Autodesk Inventor part; units mm, degrees
ref_plane "Work Plane1" through (35, 60, 0) normal (1, 0, 0) x (0, 1, 0)
ref_plane "Work Plane2" through (35, 5, 0) normal (1, 0, 0) x (0, 1, 0)
ref_plane "Work Plane3" through (35, 20, 0) normal (1, 0, 0) x (0, 1, 0)
sketch "Sketch1" plane through (0, 0, 0) normal (0, 0, 1) x (1, 0, 0)
  line L0 (0, 0) -> (0, 70)
  line L1 (0, 70) -> (-35, 70)
  line L2 (-35, 70) -> (-35, 5)
  line L3 (0, 0) -> (-32.5, 0)
  arc A0 (-35, 5) -> (-32.5, 0) centre (-28.75, 5) ccw
  dimension "d0" = 70
  dimension "d1" = 35
  dimension "d2" = 65
  dimension "d3" = 32.5
revolve "Revolution1" add sketch "Sketch1" angle 360 about axis through (0, 0, 0) along (0, 1, 0)
shell "Shell1" thickness 3 removed faces 1 at (-0.2748, 70, -9.3581)
sketch "Sketch2" plane through (0, 0, 0) normal (0, 0, 1) x (1, 0, 0)
  line L0 (35, 60) -> (60, 60)
  line L1 (35, 20) -> (64.0906, 49.6106)
  line L2 (35, 5) -> (35, 70)
  arc A0 (64.0906, 49.6106) -> (60, 60) centre (60, 54) ccw
ref_plane "Work Plane1" through (35, 60, 0) normal (1, 0, 0) x (0, 1, 0)
sketch "Sketch3" plane through (35, 60, 0) normal (1, 0, 0) x (0, 1, 0)
  ellipse E0 centre (0, 0) end of major axis (0, -6) minor radius 2
  point P0 (-60, 0)
ref_plane "Work Plane2" through (35, 5, 0) normal (1, 0, 0) x (0, 1, 0)
sketch "Sketch4" plane through (35, 5, 0) normal (1, 0, 0) x (0, 1, 0)
  point P0 (-5, 0)
ref_plane "Work Plane3" through (35, 20, 0) normal (1, 0, 0) x (0, 1, 0)
sketch "Sketch5" plane through (35, 20, 0) normal (1, 0, 0) x (0, 1, 0)
  ellipse E0 centre (0, 0) end of major axis (0, -5) minor radius 3
  point P0 (-20, 0)
sweep "Sweep1" add profiles "Sketch3" path "Sketch2" path curves L0 A0 L1
fillet "Fillet1" radius 2 2 edges at (35, 70, 0) (32, 70, 0)
sketch "Sketch6" plane through (0, 0, 0) normal (0, -1, 0) x (1, 0, 0)
  circle A0 centre (0, 0) radius 31
  circle A1 centre (0, 0) radius 32.5
  dimension "d34" = 62
  dimension "d35" = 65
extrude "Extrusion1" add sketch "Sketch6" along normal blind 2 contours A0 | A1
properties part number "Lab No. 2"
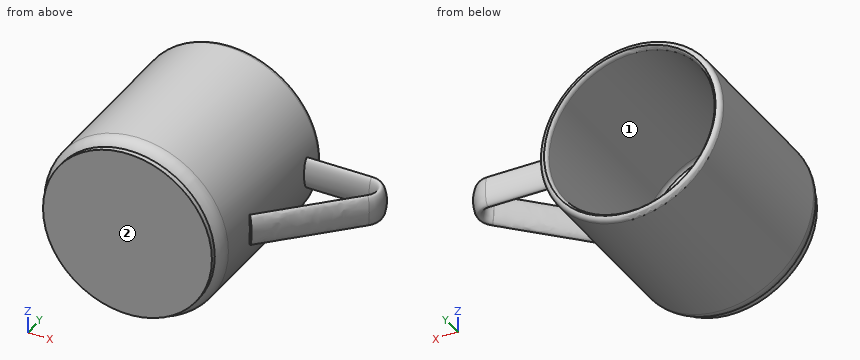
Can you work these out from the model? Positions are in its coordinate system, mm. Face numbers are marked on the shaded views. Give positions to 0.01 mm unless a question says otherwise; leave off trailing zeros. Loops run counter-clockwise (first coordinate to the right, second up) from the corner with the lowest first, then second, coordinate; pieces in that order, holes last. Notation, with made-up numbers: (84.5, 3.25) -> (121.5, 3.25) arc R27 ccw to (121.5, 37.25) -> close; hole circle Ø11 at (26.5, 89). An arc over 180 degrees is marked (long way). Return JSON: item names as keys, results as strings.
Q1. We'd pull the mould along X, two halves only. Please class the marked faces 1 and 2: released by +X, released by -X, zero draft, split by the parting line, or undercut.
Checks:
{"face 1": "undercut", "face 2": "zero draft"}
Q2. I want a section at A-A, the plane x = 0. List the corners of the cut face in (y, z) for me, then the cut area to 3 significant figures.
Checks:
{"outline": "(-2, -32.5) -> (0, -32.5) arc R6.25 ccw to (5, -35) -> (68, -35) arc R2 ccw to (70, -33) arc R2 ccw to (68.27, -32) -> (5, -32) arc R3.25 cw to (3, -31.31) -> (3, 31.31) arc R3.25 cw to (5, 32) -> (68.27, 32) arc R2 ccw to (70, 33) arc R2 ccw to (68, 35) -> (5, 35) arc R6.25 ccw to (0, 32.5) -> (-2, 32.5) -> close", "area": "733 mm2"}
Q3. For pin 1 Ø6 at (x, z) = (48, 0) entering from +Y; pin 2 Ø5 at (y, z) = (47, -2.5) entering from -X; pin 3 Ø5 at (x, y) = (-19.5, 48) entering from -Z; pin 4 Ø5 at (y, z) = (5.5, -18) entering from +X, each with a flat end and sliding along its axis, tell me the tip position at first contact or that it passes through.
Checks:
{"pin 1": "stops at y = 62", "pin 2": "stops at x = -35", "pin 3": "stops at z = -30.59", "pin 4": "stops at x = 31.38"}
Q4. I need wall thicknesses on probe 1 along Z at (x, y) = (0, 24.5); probe 2 along X at (y, z) = (47, 0); probe 3 along X at (y, z) = (30.5, 0). Which ranges of each line are inside material? Lowest first, please.
Checks:
{"probe 1": "z = -35 to -32, 32 to 35", "probe 2": "x = -35 to -32, 32 to 35, 58.72 to 64.33", "probe 3": "x = -35 to -32, 32 to 35, 42.51 to 48.12"}
Q5. I want a section at B-B, the plane y = 65. List the corners of the cut face in (x, z) for me.
Checks:
{"outline": "circle Ø70 at (0, 0); hole circle Ø64 at (0, 0)"}
Q6. I want a section at C-C, the plane y = 42.5. Count the separate pieces of the cut face and the enclosed holes in it, then the cut area to 3 significant figures.
Checks:
{"separate pieces": "2", "enclosed holes": "1", "area": "684 mm2"}
